Source: CAD feature listing. Evaluate the final solid. Frame: model axes, mm. Give positions to 0.01 mm unless a question says otherwise; leave off trailing zeros. Write each loop counter-clockwise with the first axis right and the second up, starting at its lowest first coordinate (ties: lowest second). Pieces come first, ordered by that corner, then holes. Notation, with made-up numbers: M -1.5,67.5 L 38.5,67.5 A11 cw 38.5,77.5 Z; hole C 15.5,-21 d11. An arc over 180 degrees is marked long. Answer as a JSON object with one key per item and string values. Group by question number.
```python
from build123d import *

# Parameters (mm, degrees)
BASE_FLANGE1_DEPTH = 32.004
SKETCH6_R          = 4.3688
CUT_EXTRUDE1_DEPTH = 60.723526665
SKETCH7_R          = 4.3688
CUT_EXTRUDE2_DEPTH = 60.723526665
FILLET1_R          = 3.175


# Sheet-metal steps are written as plain solids
with BuildPart() as part:
    # Sketch1 → Base-Flange1 (new body)
    with BuildSketch(Plane(origin=(0, 0, 0), x_dir=(0, 0, -1), z_dir=(1, 0, 0))):
        with BuildLine():
            Line((38.1, 0), (3.305600771, 0))
            ThreePointArc((3.305600771, 0), (0.373497077, 0.717481209), (-1.89601471, 2.707789629))
            Line((-1.89601471, 2.707789629), (-21.853262225, 31.209692887))
            Line((-21.853262225, 31.209692887), (-19.252454484, 33.030798073))
            Line((-19.252454484, 33.030798073), (0.70479303, 4.528894815))
            ThreePointArc((0.70479303, 4.528894815), (1.839548924, 3.533740605), (3.305600771, 3.175))
            Line((3.305600771, 3.175), (38.1, 3.175))
            Line((38.1, 3.175), (38.1, 0))
        make_face()
    extrude(amount=BASE_FLANGE1_DEPTH)

    # Sketch6 → Cut-Extrude1 (cut, through all)
    with BuildSketch(Plane(origin=(0, 0, 0), x_dir=(1, 0, 0), z_dir=(0, -0.5735764363510502, 0.819152044288989))):
        with Locations(Location((16.002, 25.4, 0), (0, 0, 270))):
            Circle(SKETCH6_R)
    extrude(amount=-CUT_EXTRUDE1_DEPTH, mode=Mode.SUBTRACT)

    # Sketch7 → Cut-Extrude2 (cut, through all)
    with BuildSketch(Plane.XZ):
        with Locations(Location((16.002, -25.4, 0), (0, 0, 270))):
            Circle(SKETCH7_R)
    extrude(amount=-CUT_EXTRUDE2_DEPTH, mode=Mode.SUBTRACT)

    # Fillet1
    fillet1_edges = [part.edges().sort_by_distance(p)[0] for p in [
        (32.004, 32.12024548, 20.552858355),
        (0, 32.12024548, 20.552858355),
        (32.004, 1.5875, -38.1),
        (0, 1.5875, -38.1),
    ]]
    fillet(fillet1_edges, radius=FILLET1_R)


solid = part.part
```
(1) Section B-B, the plane x = 14. Return loops of the section in (y, z) (3 decimals), plus the area to 3 significant figures.
(2) Ray query, L1, parallel to X at y = 0.65, z = -25.4; L2, parallel to Y at x = 26, z = -27.5 (3 decimals); L3, parallel to X at y = 1, z = -25. Return the intervals inside material, ascending. Write a range as [from, to].
(3) Pull-direction query (Y, two-part tool) for faces 1 (the cylindrical face through (20.334, 22.17, 13.613)), 2 (the flat face through (0, 3, -6)), 3 (the flat face through (16, 3.175, -20)), 4 (the cylindrical face through (15.78, 0.7, -0.41)); classes: pulls with the +Y half, pulls with the -Y half, needs draft (parallel to the pull), parting line crosses it, or undercut.
(4) Section D-D, the plane z = -11. Return loops of the section in (x, y) (3 decimals), plus the area to 3 significant figures.
(5) Section A-A, the plane z = -25.4. Return loops of the section in (x, y) (3 decimals).
(6) Section C-C, the plane x = 5. Return loops of the section in (y, z) (3 decimals).
(7) Contact query for flat-ended pins moving along their axis: pin 1 Ø4 at (x, z) = (20, -13) entering from +Y (3 decimals); pin 2 Ø1.5 at (x, y) = (28.5, 12) entering from -Z; pin 3 Ø5 at (x, y) = (28.5, 17.5) entering from -Z. Output: stop coordinate, or through.
Reported:
{
 "1": {"outline": "M 0,-38.1 L 3.175,-38.1 L 3.175,-29.283 L 0,-29.283 Z; M 0,-21.517 L 3.175,-21.517 L 3.175,-3.306 A3.175 cw 4.529,-0.705 L 19.447,9.741 L 17.626,12.342 L 2.708,1.896 A6.35 ccw 0,-3.306 Z; M 23.987,16.796 L 25.808,14.195 L 33.031,19.252 L 31.21,21.853 Z", "area": "186 mm2"},
 "2": {"L1": "x = [0, 11.63], [20.37, 32]", "L2": "y = [0, 3.175]", "L3": "x = [0, 11.65], [20.35, 32]"},
 "3": {"face 1": "undercut", "face 2": "needs draft", "face 3": "pulls with the +Y half", "face 4": "pulls with the -Y half"},
 "4": {"outline": "M 0,0 L 32.004,0 L 32.004,3.175 L 0,3.175 Z", "area": "102 mm2"},
 "5": {"outline": "M 0,0 L 11.633,0 L 11.633,3.175 L 0,3.175 Z; M 20.371,0 L 32.004,0 L 32.004,3.175 L 20.371,3.175 Z"},
 "6": {"outline": "M 0,-38.1 L 3.175,-38.1 L 3.175,-3.306 A3.175 cw 4.529,-0.705 L 33.031,19.252 L 31.21,21.853 L 2.708,1.896 A6.35 ccw 0,-3.306 Z"},
 "7": {"pin 1": "stops at y = 3.175", "pin 2": "stops at z = 4", "pin 3": "stops at z = 6.63"}
}
